Answer from the drawing. Dimensions are ordinates in mm from the lowest x, y and z of the part. Give positions to 0.01 mm unless a question says otherwise; leave off trailing zeros. Loops run counter-clockwise (first coordinate to the right, second up) from the corner with the lowest first, then second, coordinate; pieces in that order, holes last. Notation, with made-up numbers: (64.25, 32.5) - (71.25, 32.5) arc R29 cw to (71.25, 71.5) - close; hole circle Ø1 at (58.25, -8). An arc over 180 degrees is marked (long way). Put each result on its own line as item: value. Start each with the question number.
1. A cutting plane is placed at C-C, the plane x = 166.5. Determine the outline of the cut face in (y, z).
2. A cutting plane is placed at B-B, the plane y = 6. Determine the outline of the cut face in (x, z).
3. Given pin 1 Ø3 at (x, y) = (57.5, 4.5) entering from -Z; pin 2 Ø3 at (y, z) = (3.5, 46) entering from -X; pin 3 Ø3 at (y, z) = (5.5, 16.5) entering from -X; pin 4 Ø3 at (y, z) = (6, 12.5) entering from +X, each flat-ended and moving along its own axis, determine where each tip first touches the part or whether it passes through.
4. A cutting plane is placed at A-A, the plane z = 15. Determine the outline of the cut face in (x, y).
5. Consider L1, parallel to X at y = 5.25, z = 15; L2, parallel to X at y = 8.25, z = 6; L3, parallel to Z at x = 291.5, y = 0.5. Determine where each line is inside the solid, lowest interval first. Write a range as from..to.
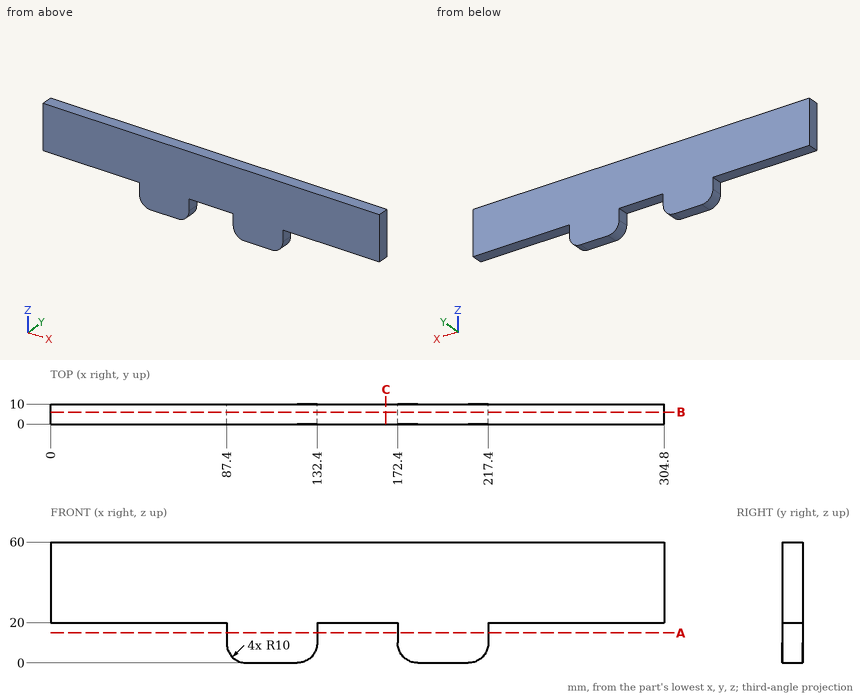
Return value:
1. outline: (0, 20) - (10, 20) - (10, 60) - (0, 60) - close
2. outline: (0, 20) - (87.4, 20) - (87.4, 10) arc R10 ccw to (97.4, 0) - (122.4, 0) arc R10 ccw to (132.4, 10) - (132.4, 20) - (172.4, 20) - (172.4, 10) arc R10 ccw to (182.4, 0) - (207.4, 0) arc R10 ccw to (217.4, 10) - (217.4, 20) - (304.8, 20) - (304.8, 60) - (0, 60) - close
3. pin 1: stops at z = 20
3. pin 2: stops at x = 0
3. pin 3: stops at x = 87.4
3. pin 4: stops at x = 217.4
4. outline: (87.4, 0) - (132.4, 0) - (132.4, 10) - (87.4, 10) - close; (172.4, 0) - (217.4, 0) - (217.4, 10) - (172.4, 10) - close
5. L1: x = 87.4..132.4, 172.4..217.4
5. L2: x = 88.23..131.57, 173.23..216.57
5. L3: z = 20..60
